from build123d import *

# Parameters (mm, degrees)
SKETCH1_R           = 5
BOSS_EXTRUDE1_DEPTH = 217.89
CUT_EXTRUDE2_DEPTH  = 105
CUT_EXTRUDE3_START  = -5
CUT_EXTRUDE3_DEPTH  = 1
FILLET1_R           = 0.2
SKETCH5_R           = 6
SKETCH5_R_2         = 5
BOSS_EXTRUDE2_DEPTH = 5
FILLET2_R           = 0.2


with BuildPart() as part:
    # Sketch1 → Boss-Extrude1 (new body)
    with BuildSketch(Plane(origin=(0, 0, 0), x_dir=(1, 0, 0), z_dir=(0, 1, 0))):
        Circle(SKETCH1_R)
    extrude(amount=BOSS_EXTRUDE1_DEPTH)

    # Sketch3 → Cut-Extrude2 (cut)
    with BuildSketch(Plane(origin=(0, 217.89, 0), x_dir=(1, 0, 0), z_dir=(0, 1, 0))):
        Polygon((3.5, 37.712556906), (3.5, 3.570714214), (3.5, -3.570714214), (3.5, -37.712556906), (71.783685384, -37.712556906), (71.783685384, 37.712556906), align=None)
    extrude(amount=-CUT_EXTRUDE2_DEPTH, mode=Mode.SUBTRACT)

    # Sketch4 → Cut-Extrude3 (cut)
    with BuildSketch(Plane(origin=(0, 217.89, 0), x_dir=(1, 0, 0), z_dir=(0, 1, 0)).offset(CUT_EXTRUDE3_START)):
        with BuildLine():
            Line((3.5, 2.666458325), (3.5, 3.570714214))
            ThreePointArc((3.5, 3.570714214), (-5, 0), (3.5, -3.570714214))
            Line((3.5, -3.570714214), (3.5, -2.666458325))
            ThreePointArc((3.5, -2.666458325), (-4.4, 0), (3.5, 2.666458325))
        make_face()
    extrude(amount=CUT_EXTRUDE3_DEPTH, mode=Mode.SUBTRACT)

    # Fillet1
    fillet1_edges = [part.edges().sort_by_distance(p)[0] for p in [
        (3.5, 212.89, -3.11858627),
        (-5, 212.89, 0),
        (3.5, 212.89, 3.11858627),
        (3.5, 213.89, -3.11858627),
        (-5, 213.89, 0),
        (3.5, 213.89, 3.11858627),
    ]]
    fillet(fillet1_edges, radius=FILLET1_R)

    # Sketch5 → Boss-Extrude2 (add)
    with BuildSketch(Plane.XZ):
        Circle(SKETCH5_R)
        Circle(SKETCH5_R_2, mode=Mode.SUBTRACT)
    extrude(amount=-BOSS_EXTRUDE2_DEPTH)

    # Fillet2
    fillet2_edges = [part.edges().sort_by_distance(p)[0] for p in [
        (-6, 5, 0),
        (-6, 0, 0),
    ]]
    fillet(fillet2_edges, radius=FILLET2_R)


solid = part.part
The listing builds one solid part. Answer for the finished solid, in the listing's coordinates (mm). A direction names the side the tool comes from. Round coordinates to 2 decimals unless told otherwise and drop trailing zeros. Order: outer loops, then holes, each group sorted by start corner. A loop starts at its lowest first (then second) coordinate and runs counter-clockwise, first axis right, second up. Notation, with made-up numbers: (50.25, -7) - (75.25, -7) arc R29 cw to (75.25, 17) - close; hole circle Ø1 at (84.5, 55). An arc over 180 degrees is marked (long way). Write item = value, one per line. Start each with the question number.
1) Section D-D, the plane y = 115 is taken. Write down the section's boundary in (x, z), plus the area to 3 significant figures.
2) Given pin 1 (1 mm diameter, centred on y = 158, z = 4, fed in from -X); pin 2 (1 mm diameter, centred on y = 149, z = 0.5, fed in from -X); pin 3 (5 mm diameter, centred on y = 138.5, z = 4, fed in from -X), each flat-ended and moving along its own axis, determine where each tip first touches the part or whether it passes through.
3) Straight lines are drawn through the part: L1, parallel to Y at x = -3, z = -3.5; L2, parallel to Y at x = 4.25, z = -2.5; L3, parallel to X at y = 168, z = -3.5. For each, find the intervals that lie inside material, in ascending order.
4) For faces 4 (the flat face through (0, 0, 0)), 5 (the flat face through (2, 5, 5)), 6 (the flat face through (3.5, 166, 0)), determine the directions among +Z, -Z, +X, -X, +Y, -Y from which every point of the face is accessible in a straight line to the end or side of a thin tool.
5) For a pull along Y with two mould halves and no side action, classify faces 1 (the cylindrical face through (-5, 107, 0)), 2 (the flat face through (-1, 217.89, 0)), 3 (the cylindrical face through (-4.397, 213.38, 0.153)) as released by +Y, released by -Y, zero draft, split by the parting line, or undercut.
6) Section A-A, the plane z = 0 is taken. Write down the section's boundary in (x, y), plus the area to 3 significant figures.
7) Section C-C, the plane y = 19.5 is taken. Write down the section's boundary in (x, z), plus the area to 3 significant figures.
8) Section B-B, the plane x = 0 is taken. Write down the section's boundary in (y, z), plus the area to 3 significant figures.
Results list:
q1.outline = (3.5, -3.57) - (3.5, 3.57) arc R5 ccw (long way) to start
q1.area = 71.2 mm^2
q2.pin_1 = -3.57
q2.pin_2 = -5
q2.pin_3 = -4.77
q3.L1 = 0 to 212.89, 213.89 to 217.89
q3.L2 = 0 to 112.89
q3.L3 = -3.57 to 3.5
q4.face_4 = +Z, -Z, +X, -X, -Y
q4.face_5 = +Y
q4.face_6 = +Z, -Z, +X, +Y
q5.face_1 = zero draft
q5.face_2 = released by +Y
q5.face_3 = undercut
q6.outline = (-6, 0.2) arc R0.2 ccw to (-5.8, 0) - (5.8, 0) arc R0.2 ccw to (6, 0.2) - (6, 4.8) arc R0.2 ccw to (5.8, 5) - (5, 5) - (5, 112.89) - (3.5, 112.89) - (3.5, 217.89) - (-5, 217.89) - (-5, 214.09) arc R0.2 ccw to (-4.8, 213.89) - (-4.4, 213.89) - (-4.4, 212.89) - (-4.8, 212.89) arc R0.2 ccw to (-5, 212.69) - (-5, 5) - (-5.8, 5) arc R0.2 ccw to (-6, 4.8) - close
q6.area = 2,030 mm^2
q7.outline = circle Ø10 at (0, 0)
q7.area = 78.5 mm^2
q8.outline = (0, -5.8) arc R0.2 ccw to (0.2, -6) - (4.8, -6) arc R0.2 ccw to (5, -5.8) - (5, -5) - (212.69, -5) arc R0.2 ccw to (212.89, -4.8) - (212.89, -4.4) - (213.89, -4.4) - (213.89, -4.8) arc R0.2 ccw to (214.09, -5) - (217.89, -5) - (217.89, 5) - (214.09, 5) arc R0.2 ccw to (213.89, 4.8) - (213.89, 4.4) - (212.89, 4.4) - (212.89, 4.8) arc R0.2 ccw to (212.69, 5) - (5, 5) - (5, 5.8) arc R0.2 ccw to (4.8, 6) - (0.2, 6) arc R0.2 ccw to (0, 5.8) - close
q8.area = 2,190 mm^2
